Here's how the part is built. I have some questions about the finished solid (model axes, mm). Coordinates: 2 decimals unless noted, no trailing zeros. Loops run counter-clockwise (first coordinate to the right, second up) from the corner with the lowest first, then second, coordinate; pieces in that order, holes last. Notation, with made-up numbers: (-19, 25) - (-12, 25) arc R29 ccw to (-12, 50) - close; hole circle Ø2 at (-17.5, -11.75). An arc over 180 degrees is marked (long way). Use a Markdown table: item, result.
```python
from build123d import *

# Parameters (mm, degrees)
SKETCH1_W           = 62
SKETCH1_H           = 106
SKETCH1_R           = 1.75
BOSS_EXTRUDE1_DEPTH = 1
SKETCH2_R           = 5
BOSS_EXTRUDE2_DEPTH = 17
FILLET1_R           = 5


with BuildPart() as part:
    # Sketch1 → Boss-Extrude1 (new body)
    with BuildSketch(Plane(origin=(0, 0, 0), x_dir=(1, 0, 0), z_dir=(0, 1, 0))):
        Rectangle(SKETCH1_W, SKETCH1_H)
        with Locations((22.5, -21.5)):
            Circle(SKETCH1_R, mode=Mode.SUBTRACT)
        with Locations((22.5, 21.5)):
            Circle(SKETCH1_R, mode=Mode.SUBTRACT)
    extrude(amount=BOSS_EXTRUDE1_DEPTH)

    # Sketch2 → Boss-Extrude2 (add)
    with BuildSketch(Plane.XZ):
        Circle(SKETCH2_R)
    extrude(amount=BOSS_EXTRUDE2_DEPTH)

    # Fillet1
    fillet1_edges = [part.edges().sort_by_distance(p)[0] for p in [
        (-5, -17, 0),
    ]]
    fillet(fillet1_edges, radius=FILLET1_R)


solid = part.part
```
Q1. I want a section at A-A, the plane z = -21.5. Write out the boundary of the cut face in (x, y), then the cut area to 3 significant figures.
Check values:
| item | result |
|---|---|
| outline | (-31, 0) - (20.75, 0) - (20.75, 1) - (-31, 1) - close; (24.25, 0) - (31, 0) - (31, 1) - (24.25, 1) - close |
| area | 58.5 mm^2 |
Q2. I want a section at B-B, the plane x = 22.5. Write out the boundary of the cut face in (y, z), then the cut area to 3 significant figures.
Check values:
| item | result |
|---|---|
| outline | (0, -53) - (1, -53) - (1, -23.25) - (0, -23.25) - close; (0, -19.75) - (1, -19.75) - (1, 19.75) - (0, 19.75) - close; (0, 23.25) - (1, 23.25) - (1, 53) - (0, 53) - close |
| area | 99.0 mm^2 |
Q3. Will this pin go through, and if not, where does the flat tip stop? P1, Ø8, axis at x = 6, y = -10, coming from the -Z side.
Check values:
| item | result |
|---|---|
| P1 | z = -4.58 |
Q4. If we mould it in two halves opening along Z, with no side actions, what happens to faces 1 (the face through (21.21, 0.49, -22.68)), 2 (the face through (-1.08, -5.92, -4.88)), 3 (the face through (0, 1, -1))? For each: pulls with the +Z half, pulls with the -Z half, needs draft (parallel to the pull), parting line crosses it, or undercut.
Check values:
| item | result |
|---|---|
| face 1 | undercut |
| face 2 | parting line crosses it |
| face 3 | needs draft |
Q5. Please list where these lines run through material, in increasing order: L1, parallel to Z at x = 22.5, y = 0.6; L2, parallel to X at y = 0.5, z = -21.5; L3, parallel to Y at x = -13, z = 17.5. Write a range as from..to.
Check values:
| item | result |
|---|---|
| L1 | -53..-23.25, -19.75..19.75, 23.25..53 |
| L2 | -31..20.75, 24.25..31 |
| L3 | 0..1 |
Q6. I want a section at D-D, the plane y = -11. Write out the boundary of the cut face in (x, z).
Check values:
| item | result |
|---|---|
| outline | circle Ø10 at (0, 0) |
Q7. I want a section at C-C, the plane x = 0. Write out the boundary of the cut face in (y, z).
Check values:
| item | result |
|---|---|
| outline | (-12, -5) - (0, -5) - (0, -53) - (1, -53) - (1, 53) - (0, 53) - (0, 5) - (-12, 5) arc R5 ccw to start |
